Autodesk Inventor part; units mm, degrees
ref_plane "작업 평면1" through (125, 0, 0) normal (-1, 0, 0) x (0, 0, 1)
ref_plane "작업 평면2" through (65, 40, 45) normal (0, 1, 0) x (1, 0, 0)
ref_plane "작업 평면3" through (125, 0, 0) normal (1, 0, 0) x (0, 0, -1)
sketch "스케치1" plane through (0, 0, 0) normal (0, 0, 1) x (1, 0, 0)
  line L0 (0, 0) -> (250, 0)
  line L1 (250, 0) -> (250, 10)
  line L2 (250, 10) -> (0, 10)
  line L3 (0, 10) -> (0, 0)
  dimension "d0" = 250
  dimension "d1" = 10
extrude "돌출1" add sketch "스케치1" along normal blind 45
ref_plane "작업 평면1" through (125, 0, 0) normal (-1, 0, 0) x (0, 0, 1)
ref_plane "작업 평면2" through (65, 40, 45) normal (0, 1, 0) x (1, 0, 0)
ref_plane "작업 평면3" through (125, 0, 0) normal (1, 0, 0) x (0, 0, -1)
sketch "스케치4" plane through (0, 10, 0) normal (0, 1, 0) x (1, 0, 0)
  line L0 (250, 0) -> (0, 0)
  line L1 (0, 0) -> (0, -45)
  line L2 (250, -45) -> (0, -45)
  line L3 (250, 0) -> (250, -45)
  circle A0 centre (120, -22.5) radius 2.6
  circle A1 centre (130, -22.5) radius 2.6
  line L4 (250, 0) -> (0, 0)
  point P0 (125, 0)
  point P1 (125, 0)
  dimension "d16" = 5.2
  dimension "d17" = 5.2
  dimension "d18" = 10
  dimension "d19" = 5
extrude "돌출4" cut sketch "스케치4" against normal through all contours A0 | A1
ref_plane "작업 평면4" through (0, 0, 22.5) normal (0, 0, -1) x (-1, 0, 0)
sketch "스케치6" plane through (0, 10, 0) normal (0, 1, 0) x (1, 0, 0)
  line L0 (250, 0) -> (250, -45)
  circle A0 centre (240, -22.5) radius 5
  point P0 (0, 0)
  point P1 (250, -22.5)
  point P2 (250, -22.5)
  dimension "d32" = 10
  dimension "d33" = 10
extrude "돌출6" cut sketch "스케치6" against normal through all
properties part number "다리-3"
Input: part model. Units: mm. Frame: model coordinates. Round coordinates to 2 decimals unless told otherwise and drop trailing zeros. Order: outer loops, then holes, each group sorted by start corner. A loop starts at its lowest first (then second) coordinate and runs counter-clockwise, first axis right, second up. Notation, with made-up numbers: (7, 82) - (43, 82) arc R14 cw to (43, 86) - close; hole circle Ø3 at (80.25, 64.5). An arc over 180 degrees is marked (long way). Answer as a JSON object with one key per item and string values. Group by question number.
(1) Cut plane B-B (z = 22.5). Return loops of the section in (x, y), then the cut area to 3 significant figures.
(2) Cut plane C-C (x = 240). Return loops of the section in (y, z).
(3) Cut plane A-A (x = 130). Return loops of the section in (y, z), then the cut area to 3 significant figures.
(4) Material intervals for probe 1 along X at (y, z) = (4, 22.5); probe 2 along Z at (x, y) = (120, 6.25); probe 3 along X at (y, z) = (8.75, 20.5), sorted ascending. Write a range as from..to.
(5) Draft query along X for faces 1 (the face through (250, 5, 22)), 2 (the face through (123, 5, 0)), 3 (the face through (132.4, 5.1, 23.5)), 4 (the face through (244.77, 5.07, 21)). Return one class per face: released by +X, released by -X, zero draft, split by the parting line, or undercut.
Here are the results:
{
 "1": {"outline": "(0, 0) - (117.4, 0) - (117.4, 10) - (0, 10) - close; (122.6, 0) - (127.4, 0) - (127.4, 10) - (122.6, 10) - close; (132.6, 0) - (235, 0) - (235, 10) - (132.6, 10) - close; (245, 0) - (250, 0) - (250, 10) - (245, 10) - close", "area": "2,300 mm^2"},
 "2": {"outline": "(0, 0) - (10, 0) - (10, 17.5) - (0, 17.5) - close; (0, 27.5) - (10, 27.5) - (10, 45) - (0, 45) - close"},
 "3": {"outline": "(0, 0) - (10, 0) - (10, 19.9) - (0, 19.9) - close; (0, 25.1) - (10, 25.1) - (10, 45) - (0, 45) - close", "area": "398 mm^2"},
 "4": {"probe 1": "x = 0..117.4, 122.6..127.4, 132.6..235, 245..250", "probe 2": "z = 0..19.9, 25.1..45", "probe 3": "x = 0..118.34, 121.66..128.34, 131.66..235.42, 244.58..250"},
 "5": {"face 1": "released by +X", "face 2": "zero draft", "face 3": "undercut", "face 4": "undercut"}
}
